Check sheet for the modelled part. Datum: model origin and axes. Units: mm. Face numbers are marked on the shaded views. A direction names the side the tool comes from. Coordinates: 2 decimals unless noted, no trailing zeros. Order: outer loops, then holes, each group sorted by start corner. A loop starts at its lowest first (then second) coordinate and runs counter-clockwise, first axis right, second up.
1. Set-up check for the marked faces 5, 6 and 7: record each of +Z, -Z, +X, -X, +Y, -Y from which the full face is reachable in a straight line by a thin tool's end or side.
2. Gauge pin test, flat ends, axial feed: pin 1 Ø1.5 at (x, y) = (-0.5, 2) entering from -Z; pin 2 Ø1.2 at (x, z) = (-0.5, 18) entering from -Y; pin 3 Ø2 at (y, z) = (-1, 11) entering from +X; pin 4 Ø1.2 at (x, z) = (0, 8.5) entering from -Y. Record the tip position at first contact, or that the pin passes through.
3. Cross-section at C-C (y = -3.5). Enter the section's corners in (x, z), then the cut area to 3 significant figures.
4. Cross-section at B-B (y = -1). Enter the section's corners in (x, z).
5. Cross-section at D-D (x = 1). Count the separate pieces of the cut face and the enclosed holes in it, then the cut area to 3 significant figures.
6. Thickness scan on line 1 (Y direction, x = -0.5, z = 19.5) (3 decimals); line 2 (Z direction, x = 0.5, y = -1); line 3 (Z direction, x = 0.9, y = -0.75). Record the ranges inside material, lowest first.
7. Draft check along Z on the marked faces 1, 2, 3 and 4. Enter one of: released by +Z, released by -Z, zero draft, split by the parting line, or undercut.
8. Cross-section at A-A (z = 3.5). Enter the section's corners in (x, y).
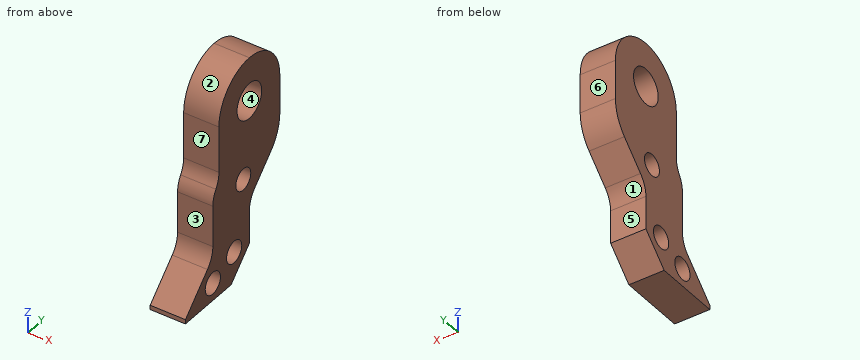
Autodesk Inventor part; units mm, degrees
ref_plane "YZ Plane" through (0, 0, 0) normal (1, 0, 0) x (0, 1, 0)
ref_plane "XZ Plane" through (0, 0, 0) normal (0, 1, 0) x (-1, 0, 0)
ref_plane "XY Plane" through (0, 0, 0) normal (0, 0, 1) x (1, 0, 0)
sketch "Skizze1" plane through (0, 0, 0) normal (1, 0, 0) x (0, 1, 0)
  line L0 (-6, 5) -> (-10.5, 0.5)
  line L1 (-10.5, 0) -> (-3, 0)
  line L2 (0, 3) -> (0, 8)
  line L3 (-10.5, 0.5) -> (-10.5, 0)
  line L4 (0, 8) -> (5, 13)
  line L5 (0, 8) -> (0, 19.5) construction
  circle A0 centre (0, 19.5) radius 0.5
  line L6 (-5, 13) -> (-5, 24.5)
  line L7 (-5, 24.5) -> (5, 24.5)
  line L8 (5, 24.5) -> (5, 13)
  line L9 (0, 3) -> (-3, 0)
  line L10 (-5, 13) -> (-6, 12)
  line L11 (-6, 12) -> (-6, 5)
  line L12 (5, 13) -> (-5, 13) construction
  point P0 (0, 0)
  point P1 (0, 0)
  dimension "d67" = 0.5
  dimension "d68" = 10.5
  dimension "d69" = 1
  dimension "d70" = 5
  dimension "d71" = 19.5
  dimension "d72" = 10
  dimension "d73" = 45
  dimension "d74" = 8
  dimension "d75" = 3
  dimension "d76" = 45
  dimension "d77" = 1
extrude "Extrusion1" add sketch "Skizze1" along normal mid plane 4
sketch "Skizze3" plane through (-2, 0, 0) normal (-1, 0, 0) x (0, 0, 1)
  line L0 (0, 8.1) -> (0, -13.6)
  circle A0 centre (19.5, 0) radius 0.5
hole "Bohrung1" at (-2, 0, 19.5) direction (1, 0, 0) diameter 4.05 end through all
sketch "Skizze4" plane through (-2, 0, 0) normal (-1, 0, 0) x (0, 0, 1)
  line L0 (-4.9, 0) -> (29.4, 0)
  line L1 (0, 8.1) -> (0, -13.6)
  point P0 (11, -1)
  dimension "d36" = 1
  dimension "d37" = 11
hole "Bohrung2" at (-2, -1, 11) direction (1, 0, 0) diameter 2.459 end through all
fillet "Rundung2" radius 5 3 edges at (0, 5, 24.5) (0, -5, 24.5) (0, 5, 13)
fillet "Rundung4" radius 3 4 edges at (0, -5, 13) (0, -6, 12) (0, 0, 8) (0, -6, 5)
sketch "Skizze5" plane through (-2, 0, 0) normal (-1, 0, 0) x (0, 0, 1)
  line L0 (-4.9, 0) -> (29.4, 0)
  line L1 (0, 8.1) -> (0, -13.6)
  point P0 (0, 0)
  point P1 (3.7, -4)
  dimension "d38" = 4
  dimension "d39" = 3.7
hole "Bohrung3" [suppressed]
sketch "Skizze6" plane through (-2, 0, 0) normal (-1, 0, 0) x (0, 0, 1)
  line L0 (-4.9, 0) -> (29.4, 0)
  line L1 (0, 8.1) -> (0, -13.6)
  circle A0 centre (3.5, -2.5) radius 1.5 construction
  circle A1 centre (2, -6) radius 1.5 construction
  line L2 (6, 0) -> (6, -6) construction
  line L3 (10.926, -6) -> (6.2426, -6) construction
  point P0 (0, 0)
  dimension "d80" = 3
  dimension "d81" = 3
  dimension "d83" = 6
  dimension "d85" = 1
  dimension "d86" = 1
  dimension "d87" = 1.5
  dimension "d88" = 3.5
hole "Bohrung4" at (-2, -6, 2) at (-2, -2.5, 3.5) direction (1, 0, 0) diameter 2.5 end through all
mirror "Spiegeln1" [suppressed]
properties part number "Chip Schaufel Seite" material "Aluminium 6061"
Data:
1. face 5: -Z, +X, -X, +Y
1. face 6: +Z, -Z, +X, -X, +Y
1. face 7: +Z, +X, -X, -Y
2. pin 1: stops at z = 9.25
2. pin 2: stops at y = -5
2. pin 3: passes through
2. pin 4: stops at y = -6
3. outline: (-2, 0) - (2, 0) - (2, 2.75) - (-2, 2.75) - close; (-2, 4.25) - (2, 4.25) - (2, 23.07) - (-2, 23.07) - close
3. area: 86.3 mm2
4. outline: (-2, 2) - (2, 2) - (2, 9.77) - (-2, 9.77) - close; (-2, 12.23) - (2, 12.23) - (2, 17.74) - (-2, 17.74) - close; (-2, 21.26) - (2, 21.26) - (2, 24.4) - (-2, 24.4) - close
5. separate pieces: 1
5. enclosed holes: 4
5. area: 175 mm2
6. line 1: y = -5 to -2.025, 2.025 to 5
6. line 2: z = 2 to 9.77, 12.23 to 17.74, 21.26 to 24.4
6. line 3: z = 2.25 to 9.8, 12.2 to 17.62, 21.38 to 24.44
7. face 1: released by -Z
7. face 2: released by +Z
7. face 3: zero draft
7. face 4: undercut
8. outline: (-2, -7.5) - (2, -7.5) - (2, -3.75) - (-2, -3.75) - close; (-2, -1.25) - (2, -1.25) - (2, 0) - (-2, 0) - close
